```python
from build123d import *

# Parameters (mm, degrees)
ESQUISSE1_W                  = 335
ESQUISSE1_H                  = 80
BOSS_EXTRU_1_DEPTH           = 5
ESQUISSE2_W                  = 5
ESQUISSE2_H                  = 80
BOSS_EXTRU_2_DEPTH           = 30
ENL_V_MAT_EXTRU_1_DEPTH      = 347.193587462
ENL_V_MAT_EXTRU_1_DEPTH_BACK = 347.193587462
ESQUISSE3_R                  = 2.25
CONG_1_R                     = 6
CONVERTIR_VOLUME2_DEPTH      = 80
CONVERTIR_VOLUME2_2_DEPTH    = 80


# Read off the part's stored shape, not the designer's step: Convertir-Volume2
with BuildPart() as part:
    # Esquisse1 → Boss.-Extru.1 (new body)
    with BuildSketch(Plane.XY):
        with Locations((167.5, 40)):
            Rectangle(ESQUISSE1_W, ESQUISSE1_H)
    extrude(amount=BOSS_EXTRU_1_DEPTH)

    # Esquisse2 → Boss.-Extru.2 (add)
    with BuildSketch(Plane.XY.offset(5)):
        with Locations((2.5, 40)):
            Rectangle(ESQUISSE2_W, ESQUISSE2_H)
        with Locations((332.5, 40)):
            Rectangle(ESQUISSE2_W, ESQUISSE2_H)
    extrude(amount=BOSS_EXTRU_2_DEPTH)

    # Esquisse3 → Enlèv. mat.-Extru.1 (cut, two sides: drawn at the far end of the back side and taken through both)
    with BuildSketch(Plane.ZY.offset(-ENL_V_MAT_EXTRU_1_DEPTH_BACK)):
        with Locations((20, 15)):
            Circle(ESQUISSE3_R)
        with Locations(Location((20, 65, 0), (0, 0, 180))):
            Circle(ESQUISSE3_R)
    extrude(amount=ENL_V_MAT_EXTRU_1_DEPTH + ENL_V_MAT_EXTRU_1_DEPTH_BACK, mode=Mode.SUBTRACT)

    # Congé1
    cong_1_edges = [part.edges().sort_by_distance(p)[0] for p in [
        (2.5, 0, 35),
        (2.5, 80, 35),
        (332.5, 0, 35),
        (332.5, 80, 35),
    ]]
    fillet(cong_1_edges, radius=CONG_1_R)

    # Convertir-Volume2 outline → Convertir-Volume2 (cut)
    with BuildSketch(Plane(origin=(0, 0, 0), x_dir=(1, 0, 0), z_dir=(0, 1, 0))):
        with BuildLine():
            ThreePointArc((0, -10), (2.928932188, -2.928932188), (10, 0))
            Line((10, 0), (0, 0))
            Line((0, 0), (0, -10))
        make_face()
        with BuildLine():
            ThreePointArc((325, 0), (332.071067812, -2.928932188), (335, -10))
            Line((335, -10), (335, 0))
            Line((335, 0), (325, 0))
        make_face()
    extrude(amount=CONVERTIR_VOLUME2_DEPTH, mode=Mode.SUBTRACT)

    # Convertir-Volume2 2 outline → Convertir-Volume2 2 (add)
    with BuildSketch(Plane(origin=(0, 0, 0), x_dir=(1, 0, 0), z_dir=(0, 1, 0))):
        with BuildLine():
            ThreePointArc((5, -10), (6.464466094, -6.464466094), (10, -5))
            Line((10, -5), (5, -5))
            Line((5, -5), (5, -10))
        make_face()
        with BuildLine():
            ThreePointArc((325, -5), (328.535533906, -6.464466094), (330, -10))
            Line((330, -10), (330, -5))
            Line((330, -5), (325, -5))
        make_face()
    extrude(amount=CONVERTIR_VOLUME2_2_DEPTH)


solid = part.part
```
CAD build for the part. Positions are in the model's coordinates, mm. A direction names the side the tool comes from. Round coordinates to 2 decimals unless told otherwise and drop trailing zeros. Write each loop counter-clockwise with the first axis right and the second up, starting at its lowest first coordinate (ties: lowest second). Pieces come first, ordered by that corner, then holes.
Item 1: Drop flat-ended pins along their axis: pin 1 Ø4 at (y, z) = (45, 5) entering from -X; pin 2 Ø1 at (x, y) = (123.5, 45) entering from +Z. Give the stop position or say it passes through.
Filled in:
pin 1: stops at x = 0.46
pin 2: stops at z = 5
Item 2: Tool access for faces 4 (the flat face through (5, 39, 22)), 5 (the cylindrical face through (2.85, 39.44, 3.01)): list every direction of +Z, -Z, +X, -X, +Y, -Y with a clear straight run to the whole face (end or side of a thin tool).
Filled in:
face 4: +Z, +Y, -Y
face 5: -Z, -X, +Y, -Y
Item 3: Band-saw the part on B-B on y = 58.5. Write the cut outline in (x, z).
Filled in:
outline: (0, 10) arc R10 ccw to (10, 0) - (325, 0) arc R10 ccw to (335, 10) - (335, 35) - (330, 35) - (330, 10) arc R5 cw to (325, 5) - (10, 5) arc R5 cw to (5, 10) - (5, 35) - (0, 35) - close
Item 4: Drill centre lines: L1, parallel to Y at x = 331, z = 20; L2, parallel to X at y = 25, z = 22.5; L3, parallel to Z at x = 222, y = 60. Where is each one in solid material? Low to high.
Filled in:
L1: y = 0 to 12.75, 17.25 to 62.75, 67.25 to 80
L2: x = 0 to 5, 330 to 335
L3: z = 0 to 5
Item 5: Mould opens along X. For faces 1 (the flat face through (0, 39, 22)), 2 (the flat face through (335, 39, 22)), 3 (the flat face through (330, 39, 22)) say: released by +X, released by -X, zero draft, split by the parting line, or undercut.
Filled in:
face 1: released by -X
face 2: released by +X
face 3: undercut
Item 6: Band-saw the part on C-C on x = 301. Write the cut outline in (y, z), then the cut area to 3 significant figures.
Filled in:
outline: (0, 0) - (80, 0) - (80, 5) - (0, 5) - close
area: 400 mm2
Item 7: Band-saw the part on A-A on z = 14.5. Write the cut outline in (x, y).
Filled in:
outline: (0, 0) - (5, 0) - (5, 80) - (0, 80) - close; (330, 0) - (335, 0) - (335, 80) - (330, 80) - close
